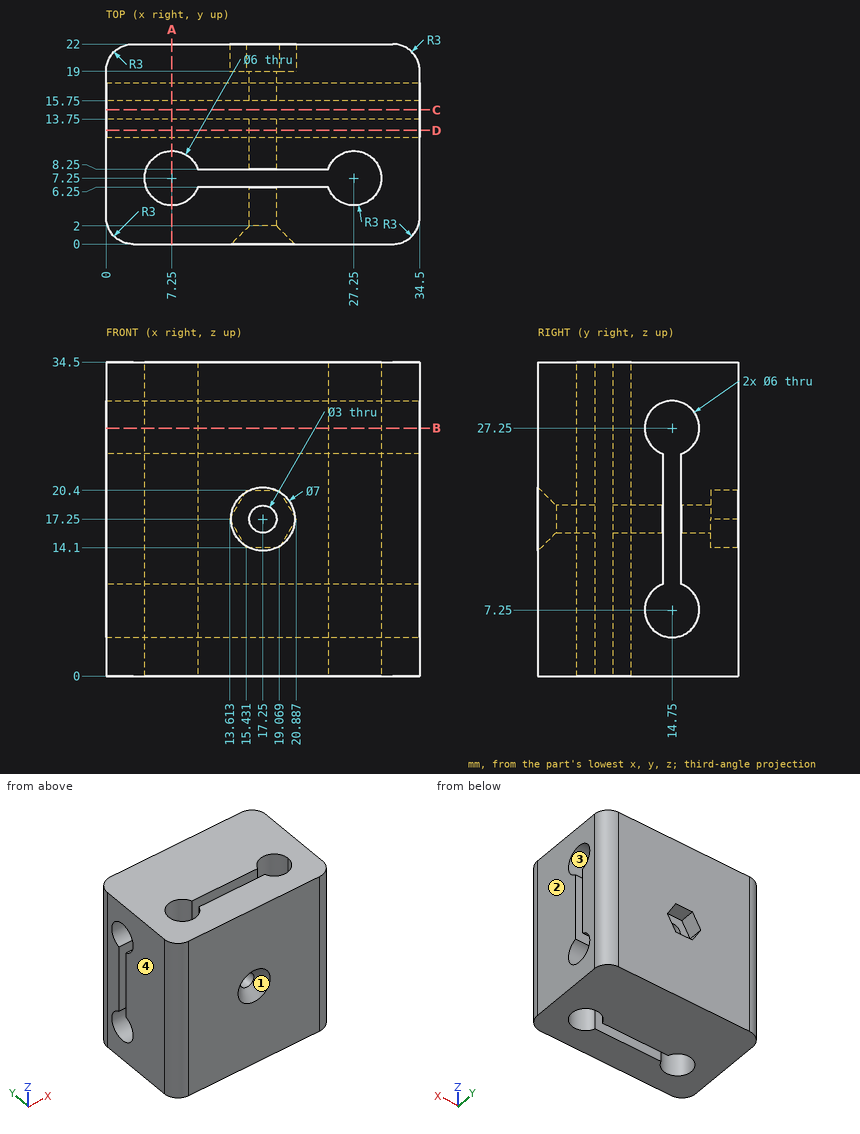
Design review of the part shown in the three views and the two pictorial views. Dimensions are in mm from the part's minimum x, y and z. Give positions to 0.01 mm unless a question says otherwise; leave off trailing zeros. Loops run counter-clockwise (first coordinate to the right, second up) from the corner with the lowest first, then second, coordinate; pieces in that order, holes last. Notation, with made-up numbers: M 76,-15 L 112,-15 A20 cw 112,4 Z; hole C 73.25,13.25 d5. An arc over 180 degrees is marked long. Write item = value, one per line.
Q1. To check wall thickness, follow line 1 (Y direction, x = 16, z = 7); line 2 (Y direction, x = 26, z = 17.5); line 3 (X direction, y = 17.55, z = 17.25). State the ranges of each line that lie inside material, in increasing order. Write a range as [from, to].
Output values:
line_1 = [0, 6.25], [8.25, 11.76], [17.74, 22]
line_2 = [0, 4.52], [9.98, 13.75], [15.75, 22]
line_3 = [0, 15.75], [18.75, 34.5]
Q2. We need section A-A (x = 7.25). Give the boundary of the cut face in (y, z), plus the area to 3 significant figures.
Output values:
outline = M 0,0 L 4.25,0 L 4.25,34.5 L 0,34.5 Z; M 10.25,0 L 22,0 L 22,34.5 L 10.25,34.5 Z; hole M 13.75,10.08 A3 ccw long 15.75,10.08 L 15.75,24.42 A3 ccw long 13.75,24.42 Z
area = 467 mm^2
Q3. Draft analysis for pull direction X (two halves, no side actions). For the marked faces 1, 2, 3 and 4, state which applies: +X half, -X half, draft (parallel to the pull), parting line (faces both ways), or undercut.
Output values:
face_1 = undercut
face_2 = +X half
face_3 = draft
face_4 = -X half
Q4. We need section B-B (z = 27.25). Give the boundary of the cut face in (x, y).
Output values:
outline = M 0,3 A3 ccw 3,0 L 31.5,0 A3 ccw 34.5,3 L 34.5,11.75 L 0,11.75 Z; M 0,17.75 L 34.5,17.75 L 34.5,19 A3 ccw 31.5,22 L 3,22 A3 ccw 0,19 Z; hole M 10.08,6.25 L 24.42,6.25 A3 ccw long 24.42,8.25 L 10.08,8.25 A3 ccw long Z
Q5. We need section D-D (y = 12.5). Count the separate pieces of the cut face and the enclosed holes in it.
Output values:
separate_pieces = 3
enclosed_holes = 1
Q6. We need section C-C (y = 14.75). Give the boundary of the cut face in (x, z).
Output values:
outline = M 0,0 L 34.5,0 L 34.5,4.25 L 0,4.25 Z; M 0,30.25 L 34.5,30.25 L 34.5,34.5 L 0,34.5 Z
Q7. Insertion check: pin 1 (5 mm diameter, centred on x = 17.25, z = 17.25, fed in from -Y); pin 2 (5 mm diameter, centred on x = 17.25, z = 17.25, fed in from +Y). Each pin has a flat end and moves straight along its axis. Give the tip position at first contact, or say it passes through.
Output values:
pin_1 = 1
pin_2 = 19
